For this review, take the finished solid that the model builds, in its own axes (mm). Face numbers are marked on the shaded views. A direction names the side the tool comes from. Give positions to 0.01 mm unless a question says otherwise; leave off trailing zeros. Order: outer loops, then holes, each group sorted by start corner. A loop starts at its lowest first (then second) coordinate and runs counter-clockwise, first axis right, second up.
from build123d import *

# Parameters (mm, degrees)
F0_R     = 38.1
F0_R_2   = 6.35
F0_R_3   = 12.7
F1_DEPTH = 8.89
F2_SIZE  = 1.27
F3_DEPTH = 25.4
F4_R     = 7.47533
F5_DEPTH = 173.482


with BuildPart() as f1:
    # F0 (on Top) → F1 (new body)
    with BuildSketch(Plane.XY):
        Circle(F0_R)
        with Locations((0, -25.4)):
            Circle(F0_R_2, mode=Mode.SUBTRACT)
        with Locations((-25.4, 0)):
            Circle(F0_R_2, mode=Mode.SUBTRACT)
        Circle(F0_R_3, mode=Mode.SUBTRACT)
        with Locations((25.4, 0)):
            Circle(F0_R_2, mode=Mode.SUBTRACT)
        with Locations((0, 25.4)):
            Circle(F0_R_2, mode=Mode.SUBTRACT)
    extrude(amount=F1_DEPTH)

    # F2
    f2_edges = [f1.edges().sort_by_distance(p)[0] for p in [
        (-38.1, 0, 8.89),
    ]]
    chamfer(f2_edges, length=F2_SIZE)

    # F0 (on Top) → F3 (join)
    with BuildSketch(Plane.XY):
        Circle(F0_R_3)
    extrude(amount=F3_DEPTH)

    # F4 (on Top) → F5 (cut)
    with BuildSketch(Plane.XY):
        Circle(F4_R)
    extrude(amount=F5_DEPTH, mode=Mode.SUBTRACT)


solid = f1.part
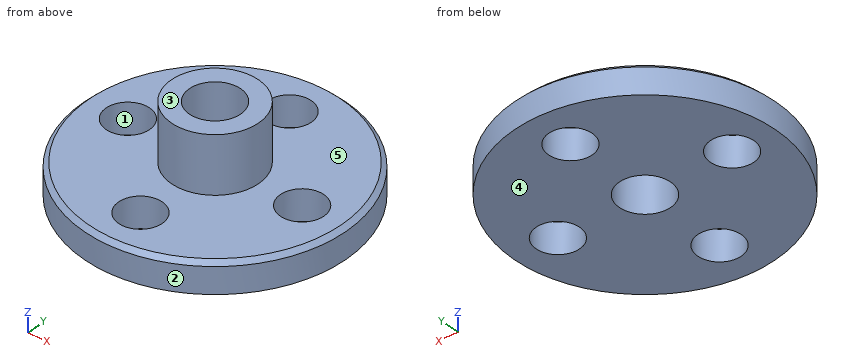
1) Draft analysis for pull direction X (two halves, no side actions). For the marked faces 1, 2 and 3, state which applies: +X half, -X half, draft (parallel to the pull), parting line (faces both ways), or undercut.
Answer sheet:
face 1: undercut
face 2: parting line
face 3: draft
2) We need section A-A on x = 0. Give the boundary of the cut face in (y, z), then the cut area to 3 significant figures.
Answer sheet:
outline: (-38.1, 0) - (-31.75, 0) - (-31.75, 8.89) - (-36.83, 8.89) - (-38.1, 7.62) - close; (-19.05, 0) - (-7.48, 0) - (-7.48, 25.4) - (-12.7, 25.4) - (-12.7, 8.89) - (-19.05, 8.89) - close; (7.48, 0) - (19.05, 0) - (19.05, 8.89) - (12.7, 8.89) - (12.7, 25.4) - (7.48, 25.4) - close; (31.75, 0) - (38.1, 0) - (38.1, 7.62) - (36.83, 8.89) - (31.75, 8.89) - close
area: 490 mm2
3) Tool access review of the marked faces 4 and 5: name each direction out of +Z, -Z, +X, -X, +Y, -Y from which nothing blocks a thin tool from reaching the whole face with its end or side.
Answer sheet:
face 4: -Z, +X, -X, +Y, -Y
face 5: +Z
4) We need section D-D on z = 14. Give the boundary of the cut face in (x, y), then the cut area to 3 significant figures.
Answer sheet:
outline: circle Ø25.4 at (0, 0); hole circle Ø14.95 at (0, 0)
area: 331 mm2
5) Clearance check with flat-ended pins moving along their axes: pin 1 (12 mm diameter, centred on y = 9.5, z = 5, fed in from -X); pin 2 (1 mm diameter, centred on x = -1.5, z = 8.5, fed in from -Y); pin 3 (12 mm diameter, centred on y = -14, z = 6, fed in from +X); pin 4 (7.5 mm diameter, centred on x = -25.4, y = 0, fed in from +Z). State where each tip first meets the part, or that it passes through.
Answer sheet:
pin 1: stops at x = -37.94
pin 2: stops at y = -37.69
pin 3: stops at x = 37.25
pin 4: passes through
6) To check wall thickness, follow line 1 (Y direction, x = 0, z = 6.5); line 2 (Y direction, x = 0, z = 9.25); line 3 (Z direction, x = -23, y = 6). State the ranges of each line that lie inside material, in increasing order.
Answer sheet:
line 1: y = -38.1 to -31.75, -19.05 to -7.48, 7.48 to 19.05, 31.75 to 38.1
line 2: y = -12.7 to -7.48, 7.48 to 12.7
line 3: z = 0 to 8.89
7) We need section C-C on z = 5.5. Give the boundary of the cut face in (x, y), then the cut area to 3 significant figures.
Answer sheet:
outline: circle Ø76.2 at (0, 0); hole circle Ø12.7 at (-25.4, 0); hole circle Ø14.95 at (0, 0); hole circle Ø12.7 at (0, -25.4); hole circle Ø12.7 at (0, 25.4); hole circle Ø12.7 at (25.4, 0)
area: 3,880 mm2
